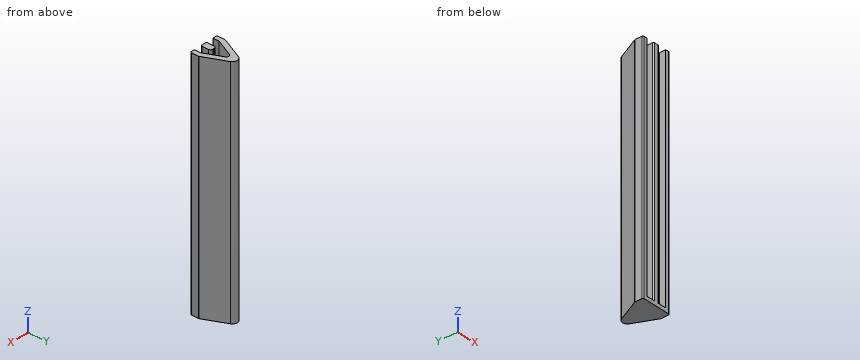
from build123d import *

# Parameters (mm, degrees)
F1_DEPTH = 1.5
F2_DEPTH = 95
F3_R     = 0.5


# Not quite as in the source:
# - a feature names something its author has since deleted; it is built from what else it names


with BuildPart() as f1:
    # F0 (on Top) → F1 (new body)
    with BuildSketch(Plane.XY):
        with BuildLine():
            ThreePointArc((0.906307787, -1.9435833214), (0, -1.3662015832), (-0.906307787, -1.9435833214))
            Line((-0.906307787, -1.9435833214), (-4.2261826174, -9.0630778704))
            Line((-4.2261826174, -9.0630778704), (-4.2261826174, -11.5630778704))
            Line((-4.2261826174, -11.5630778704), (-1.25, -11.5630778704))
            Line((-1.25, -11.5630778704), (-1.25, -8.5630778704))
            ThreePointArc((-1.25, -8.5630778704), (-0.9571067812, -7.8559710892), (-0.25, -7.5630778704))
            Line((-0.25, -7.5630778704), (0.25, -7.5630778704))
            ThreePointArc((0.25, -7.5630778704), (0.9571067812, -7.8559710892), (1.25, -8.5630778704))
            Line((1.25, -8.5630778704), (1.25, -11.5630778704))
            Line((1.25, -11.5630778704), (4.2261826174, -11.5630778704))
            Line((4.2261826174, -11.5630778704), (4.2261826174, -9.0630778704))
            Line((4.2261826174, -9.0630778704), (0.906307787, -1.9435833214))
        make_face()
        with BuildLine():
            Line((-4.2261826174, -9.0630778704), (-0.906307787, -1.9435833214))
            ThreePointArc((-0.906307787, -1.9435833214), (0, -1.3662015832), (0.906307787, -1.9435833214))
            Line((0.906307787, -1.9435833214), (4.2261826174, -9.0630778704))
            Line((4.2261826174, -9.0630778704), (4.2261826174, -11.5630778704))
            Line((4.2261826174, -11.5630778704), (6.0387981915, -11.5630778704))
            Line((6.0387981915, -11.5630778704), (6.0387981915, -8.2178413469))
            Line((6.0387981915, -8.2178413469), (1.8126155741, 0.8452365235))
            ThreePointArc((1.8126155741, 0.8452365235), (0, 2), (-1.8126155741, 0.8452365235))
            Line((-1.8126155741, 0.8452365235), (-6.0387981915, -8.2178413469))
            Line((-6.0387981915, -8.2178413469), (-6.0387981915, -11.5630778704))
            Line((-6.0387981915, -11.5630778704), (-4.2261826174, -11.5630778704))
            Line((-4.2261826174, -11.5630778704), (-4.2261826174, -9.0630778704))
        make_face()
        with BuildLine():
            Line((-1.25, -8.5630778704), (-1.25, -11.5630778704))
            Line((-1.25, -11.5630778704), (1.25, -11.5630778704))
            Line((1.25, -11.5630778704), (1.25, -8.5630778704))
            ThreePointArc((1.25, -8.5630778704), (0.9571067812, -7.8559710892), (0.25, -7.5630778704))
            Line((0.25, -7.5630778704), (-0.25, -7.5630778704))
            ThreePointArc((-0.25, -7.5630778704), (-0.9571067812, -7.8559710892), (-1.25, -8.5630778704))
        make_face()
    extrude(amount=F1_DEPTH)

    # F0 (on Top) → F2 (join)
    with BuildSketch(Plane.XY):
        with BuildLine():
            Line((-4.2261826174, -9.0630778704), (-0.906307787, -1.9435833214))
            ThreePointArc((-0.906307787, -1.9435833214), (0, -1.3662015832), (0.906307787, -1.9435833214))
            Line((0.906307787, -1.9435833214), (4.2261826174, -9.0630778704))
            Line((4.2261826174, -9.0630778704), (4.2261826174, -11.5630778704))
            Line((4.2261826174, -11.5630778704), (6.0387981915, -11.5630778704))
            Line((6.0387981915, -11.5630778704), (6.0387981915, -8.2178413469))
            Line((6.0387981915, -8.2178413469), (1.8126155741, 0.8452365235))
            ThreePointArc((1.8126155741, 0.8452365235), (0, 2), (-1.8126155741, 0.8452365235))
            Line((-1.8126155741, 0.8452365235), (-6.0387981915, -8.2178413469))
            Line((-6.0387981915, -8.2178413469), (-6.0387981915, -11.5630778704))
            Line((-6.0387981915, -11.5630778704), (-4.2261826174, -11.5630778704))
            Line((-4.2261826174, -11.5630778704), (-4.2261826174, -9.0630778704))
        make_face()
        with BuildLine():
            Line((-1.25, -8.5630778704), (-1.25, -11.5630778704))
            Line((-1.25, -11.5630778704), (1.25, -11.5630778704))
            Line((1.25, -11.5630778704), (1.25, -8.5630778704))
            ThreePointArc((1.25, -8.5630778704), (0.9571067812, -7.8559710892), (0.25, -7.5630778704))
            Line((0.25, -7.5630778704), (-0.25, -7.5630778704))
            ThreePointArc((-0.25, -7.5630778704), (-0.9571067812, -7.8559710892), (-1.25, -8.5630778704))
        make_face()
    extrude(amount=F2_DEPTH)

    # F3
    f3_edges = [f1.edges().sort_by_distance(p)[0] for p in [
        (-6.038798, -8.217841, 47.5),
        (-6.038798, -11.563078, 47.5),
        (6.038798, -8.217841, 47.5),
        (6.038798, -11.563078, 47.5),
        (-1.25, -11.563078, 48.25),
        (1.25, -11.563078, 48.25),
    ]]
    fillet(f3_edges, radius=F3_R)


solid = f1.part
Part model, mm, in its own coordinate system. Give positions to 0.01 mm unless a question says otherwise; leave off trailing zeros. Loops run counter-clockwise (first coordinate to the right, second up) from the corner with the lowest first, then second, coordinate; pieces in that order, holes last. Notation, with made-up numbers: M 19,-29 L 40,-29 A11 ccw 40,-16 Z; hole C 24,88.5 d1. An arc over 180 degrees is marked long. Put each result on its own line as item: value. Start each with the question number.
1) Saw through at C-C (y = -2.75). List the corners of the cut face in (x, z), then the cut area to 3 significant figures.
2) Flat gauge pins, fed straight in: pin 1 (1.5 mm diameter, centred on y = -6.5, z = 55, fed in from -X); pin 2 (3 mm diameter, centred on y = 0, z = 78.5, fed in from +X). Where does each tip first touch, or does it go through?
3) Saw through at A-A (z = 65). List the corners of the cut face in (x, y), then the cut area to 3 significant figures.
4) Saw through at B-B (y = -10). List the corners of the cut face in (x, z).
5) Probe probe 1 along X at (y, z) = (-10.25, 86); probe 2 along X at (y, z) = (-8.5, 51); probe 3 along Y at (x, z) = (-0.5, 12.5). List the from-to ranges inside material, lowest first.
Numbers:
1. outline: M -3.49,0 L 3.49,0 L 3.49,95 L 1.28,95 L 1.28,1.5 L -1.28,1.5 L -1.28,95 L -3.49,95 Z
1. area: 423 mm^2
2. pin 1: x = -5.59
2. pin 2: x = 2.91
3. outline: M -6.04,-11.06 A0.5 ccw -5.54,-11.56 L -4.23,-11.56 L -4.23,-9.06 L -0.91,-1.94 A1 cw 0.91,-1.94 L 4.23,-9.06 L 4.23,-11.56 L 5.54,-11.56 A0.5 ccw 6.04,-11.06 L 6.04,-8.33 A0.5 ccw 5.99,-8.12 L 1.81,0.85 A2 ccw -1.81,0.85 L -5.99,-8.12 A0.5 ccw -6.04,-8.33 Z; M -1.25,-11.06 A0.5 ccw -0.75,-11.56 L 0.75,-11.56 A0.5 ccw 1.25,-11.06 L 1.25,-8.56 A1 ccw 0.25,-7.56 L -0.25,-7.56 A1 ccw -1.25,-8.56 Z
3. area: 65.5 mm^2
4. outline: M -6.04,0 L 6.04,0 L 6.04,95 L 4.23,95 L 4.23,1.5 L 1.25,1.5 L 1.25,95 L -1.25,95 L -1.25,1.5 L -4.23,1.5 L -4.23,95 L -6.04,95 Z
5. probe 1: -6.04 to -4.23, -1.25 to 1.25, 4.23 to 6.04
5. probe 2: -6.04 to -3.96, -1.25 to 1.25, 3.96 to 6.04
5. probe 3: -11.56 to -7.59, -1.5 to 1.94
